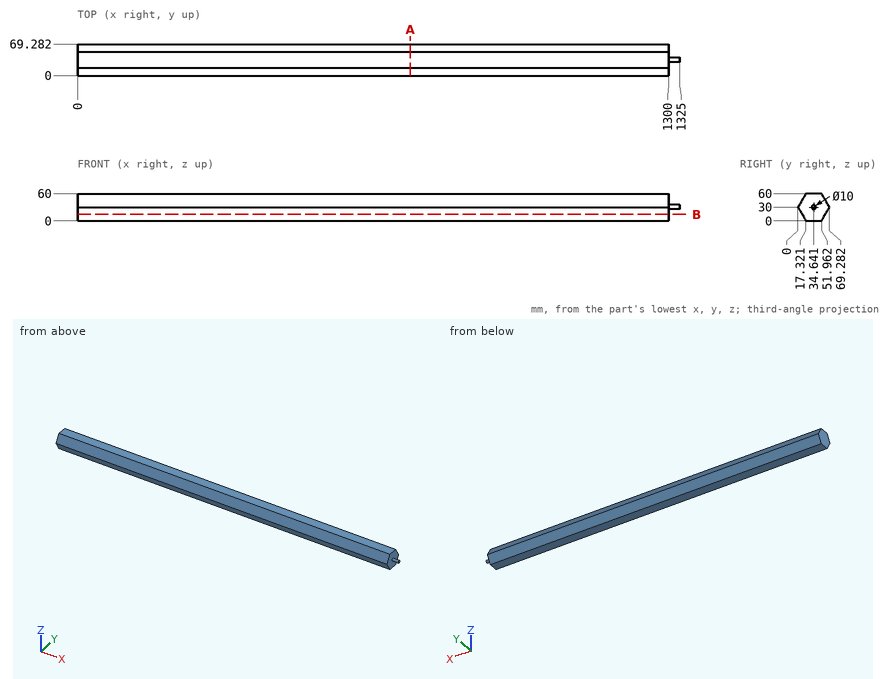
Input: dimensioned drawing with shaded views. Units: mm. Origin: part minimum x, y, z. Round coordinates to 2 decimals unless told otherwise and drop trailing zeros. Loops run counter-clockwise (first coordinate to the right, second up) from the corner with the lowest first, then second, coordinate; pieces in that order, holes last. Notation, with made-up numbers: (2.5, 79) -> (45.5, 79) arc R15 cw to (45.5, 91) -> close; hole circle Ø6 at (-1.75, 40.25). An arc over 180 degrees is marked (long way). Answer as a JSON object with one key per item and string values. Group by question number.
Q1. Contact query for flat-ended pins moving along their axis: P1, Ø2, axis at y = 36, z = 46, coming from the +X side; P2, Ø1, axis at x = 164.5, z = 23.5, coming from the +Y side; P3, Ø1, axis at x = 652, z = 36, coming from the -Y side (1 decimal). Output: stop coordinate, or through.
Q2. Section query A-A (x = 732). Output: boundary loops of the cut face in (y, z), plus the area to 3 significant figures.
Q3. Ray query, line 1 (X direction, y = 64, z = 29); line 2 (Y direction, x = 645, z = 54.5) (1 decimal); line 3 (Y direction, x = 418, z = 57) (1 decimal). Return the intervals inside material, ascending. Write a range as from..to.
Q4. Section query B-B (z = 14). Output: boundary loops of the cut face in (x, y) (1 decimal).
Completed:
{
 "1": {"P1": "x = 1300", "P2": "y = 65.82", "P3": "y = 3.2"},
 "2": {"outline": "(0, 30) -> (17.32, 0) -> (51.96, 0) -> (69.28, 30) -> (51.96, 60) -> (17.32, 60) -> close", "area": "3,120 mm²"},
 "3": {"line 1": "0..1300", "line 2": "14.1..55.1", "line 3": "15.6..53.7"},
 "4": {"outline": "(0, 9.2) -> (1300, 9.2) -> (1300, 60) -> (0, 60) -> close"}
}
